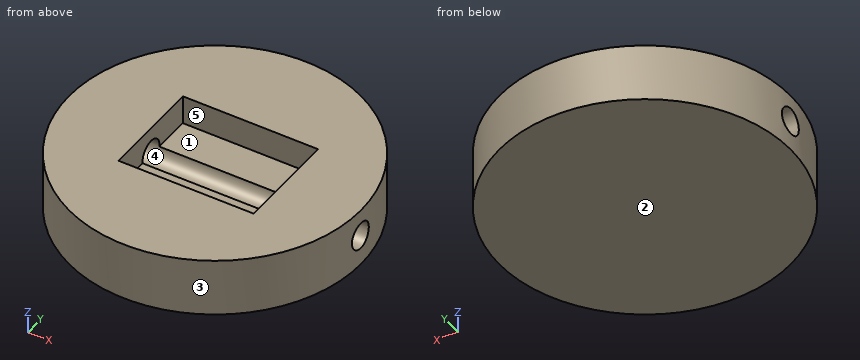
from build123d import *

# Parameters (mm, degrees)
F0_R     = 63.5
F1_DEPTH = 25.4
F2_W     = 58.809195
F2_H     = 44.798226
F3_DEPTH = 12.7
F4_R     = 5.867583
F5_DEPTH = 127


with BuildPart() as f1:
    # F0 (on Top) → F1 (new body)
    with BuildSketch(Plane.XY):
        Circle(F0_R)
    extrude(amount=F1_DEPTH)

    # F2 (on face) → F3 (cut)
    with BuildSketch(Plane.XY.offset(25.4)):
        with Locations((1.567016, -0.276532)):
            Rectangle(F2_W, F2_H)
    extrude(amount=-F3_DEPTH, mode=Mode.SUBTRACT)

    # F4 (on Right) → F5 (cut, symmetric)
    with BuildSketch(Plane.YZ):
        with Locations((0, 13.457903)):
            Circle(F4_R)
    extrude(amount=F5_DEPTH, both=True, mode=Mode.SUBTRACT)


solid = f1.part
Source: CAD feature listing. Evaluate the final solid. Frame: model axes, mm. Face numbers are marked on the shaded views. A direction names the side the tool comes from. Give positions to 0.01 mm unless a question says otherwise; leave off trailing zeros. Loops run counter-clockwise (first coordinate to the right, second up) from the corner with the lowest first, then second, coordinate; pieces in that order, holes last. Notation, with made-up numbers: (-24, -21.75) -> (-17, -21.75) arc R15 cw to (-17, -7.75) -> close; hole circle Ø1 at (75.5, -30.5). An arc over 180 degrees is marked (long way). Use a Markdown table: item, result. Add a question column.
1) Section query A-A, the plane y = 0. Return the cut outline in (x, z), then the cut area to 3 significant figures.
2) Section query B-B, the plane z = 15.5. Return the cut outline in (x, y), then the cut area to 3 significant figures.
3) Reachability of the marked faces 4 and 5 from +Z, -Z, +X, -X, +Y, -Y: full face, straight path, thin tool, end or side. Return the list, or none.
4) Section query D-D, the plane x = -39. Return the cut outline in (y, z), then the cut area to 3 significant figures.
5) Section query C-C, the plane x = 0. Return the cut outline in (y, z).
6) Pull-direction query (Y, two-part tool) for the marked faces 1, 2 and 3; classes: +Y half, -Y half, draft (parallel to the pull), parting line (faces both ways), or undercut.
7) Line query: line 1 along Z through (x, y) = (-12, 0); line 2 along Z through (x, y) = (34, 0); line 3 along Y through (x, z) = (-23, 15). Output: solid intervals per line, ascending. Write a range as [from, to].
8) First-contact query: pin 1 (14 mm diameter, centred on y = 1, z = 17, fed in from +X); pin 2 (3 mm diameter, centred on x = -45, z = 7, fed in from -Y); pin 3 (8 mm diameter, centred on x = 29, z = 18.5, fed in from -Y); pin 4 (8 mm diameter, centred on y = -4, z = 13, fed in from +X) (3 decimals). Flat tips, straight axial feed; report the tip coordinate or a pass-through.
Numbers:
| question | item | result |
|---|---|---|
| 1 | outline | (-63.5, 0) -> (63.5, 0) -> (63.5, 7.59) -> (-63.5, 7.59) -> close; (-63.5, 19.33) -> (-27.84, 19.33) -> (-27.84, 25.4) -> (-63.5, 25.4) -> close; (30.97, 19.33) -> (63.5, 19.33) -> (63.5, 25.4) -> (30.97, 25.4) -> close |
| 1 | area | 1,380 mm2 |
| 2 | outline | (-63.26, -5.5) arc R63.5 ccw to (63.26, -5.5) -> (30.97, -5.5) -> (30.97, -22.68) -> (-27.84, -22.68) -> (-27.84, -5.5) -> close; (-63.26, 5.5) -> (-27.84, 5.5) -> (-27.84, 22.12) -> (30.97, 22.12) -> (30.97, 5.5) -> (63.26, 5.5) arc R63.5 ccw to start |
| 2 | area | 9,280 mm2 |
| 3 | face 4 | +X, -X |
| 3 | face 5 | +Z |
| 4 | outline | (-50.11, 0) -> (50.11, 0) -> (50.11, 25.4) -> (-50.11, 25.4) -> close; hole circle Ø11.74 at (0, 13.46) |
| 4 | area | 2,440 mm2 |
| 5 | outline | (-63.5, 0) -> (63.5, 0) -> (63.5, 25.4) -> (22.12, 25.4) -> (22.12, 12.7) -> (5.82, 12.7) arc R5.87 cw to (-5.82, 12.7) -> (-22.68, 12.7) -> (-22.68, 25.4) -> (-63.5, 25.4) -> close |
| 6 | face 1 | undercut |
| 6 | face 2 | draft |
| 6 | face 3 | parting line |
| 7 | line 1 | z = [0, 7.59] |
| 7 | line 2 | z = [0, 7.59], [19.33, 25.4] |
| 7 | line 3 | y = [-59.19, -22.68], [22.12, 59.19] |
| 8 | pin 1 | stops at x = 63.5 |
| 8 | pin 2 | stops at y = -46.26 |
| 8 | pin 3 | stops at y = -58.37 |
| 8 | pin 4 | stops at x = 63.385 |
